CAD build for the part. Positions are in the model's coordinates, mm. A direction names the side the tool comes from. Coordinates: 2 decimals unless noted, no trailing zeros. Order: outer loops, then holes, each group sorted by start corner. A loop starts at its lowest first (then second) coordinate and runs counter-clockwise, first axis right, second up. Notation, with made-up numbers: (-11.75, -37) - (45.25, -37) arc R15 cw to (45.25, -31) - close; hole circle Ø3 at (80.25, 57). An arc over 180 degrees is marked (long way). Write each question's results on one line, items separated by ' | '. Start each with the question number.
Q1. Pin check, flat tips, straight feed: P1, Ø4, axis at x = 12, z = 5, coming from the +Y side; P2, Ø3.5, axis at x = 2, y = 20, coming from the +Z side; P3, Ø6, axis at x = -1, y = 26.5, coming from the -Z side; P4, Ø5, axis at x = -20, y = -1.5, coming from the -Z side. Stop position of each tip, or through.
Q2. Band-saw the part on B-B, the plane z = 2.75. Write the cut outline in (x, y).
Q3. Pull direction X, two halves, no side cores. Call faces 1 (the flat face through (15.968, -2.936, 6.726)), 2 (the flat face through (10.597, -12.391, 6.726)), 3 (the flat face through (-4.28, 25.19, 3.52)): released by +X, released by -X, zero draft, split by the parting line, or undercut.
Q4. Wall check: probe 1 along Y at (x, z) = (0, 1.5); probe 2 along Y at (x, z) = (6, 5.5); probe 3 along X at (y, z) = (-15, 5). Give the ranges that are in metal, low to high.
Q5. Which spindle directions (+Z, -Z, +X, -X, +Y, -Y) get a long thin tool onto all of the face, cutting with end or side? Do faces 4 (the flat face through (11, 2, 0)), 5 (the flat face through (-19.677, -16.304, 3.517)), 6 (the flat face through (4.304, 24.995, 3.517)), 7 (the flat face through (16.03, -2.98, 0.38)), 8 (the flat face through (-16.03, -2.98, 6.73)). Say none if no direction does.
Q6. Band-saw the part on C-C, the plane y = -9. Write the cut outline in (x, z), then the cut area to 3 significant figures.
Q7. Band-saw the part on D-D, the plane x = -7. Write the cut outline in (y, z), then the cut area to 3 significant figures.
Q8. Band-saw the part on A-A, the plane x = 0. Write the cut outline in (y, z).
```python
from build123d import *

# Parameters (mm, degrees)
F0_R     = 10.922
F1_DEPTH = 7.112
F2_DEPTH = 6.35
F3_DEPTH = 0.762
F4_DEPTH = 7.112


with BuildPart() as f1:
    # F0 (on Top) → F1 (new body)
    with BuildSketch(Plane.XY):
        with BuildLine():
            Line((-5.7560840378, 12.6157379826), (-5.1183423957, 18.0540294813))
            Line((-5.1183423957, 18.0540294813), (-9.9884684203, 9.6187237673))
            ThreePointArc((-9.9884684203, 9.6187237673), (-8.0136294261, 11.3168499026), (-5.7560840378, 12.6157379826))
        make_face()
        with BuildLine():
            ThreePointArc((5.7560840378, 12.6157379826), (0, 13.8668434871), (-5.7560840378, 12.6157379826))
            ThreePointArc((-5.7560840378, 12.6157379826), (-8.0136294261, 11.3168499026), (-9.9884684203, 9.6187237673))
            Line((-9.9884684203, 9.6187237673), (-13.3242933447, 3.8409055132))
            ThreePointArc((-13.3242933447, 3.8409055132), (-13.8074942195, 1.2815817082), (-13.8035915993, -1.3229539883))
            ThreePointArc((-13.8035915993, -1.3229539883), (-12.0090387301, -6.9334217436), (-8.0475075615, -11.2927839943))
            ThreePointArc((-8.0475075615, -11.2927839943), (-5.7938647934, -12.5984316108), (-3.3358249243, -13.4596292806))
            Line((-3.3358249243, -13.4596292806), (3.3358249243, -13.4596292806))
            ThreePointArc((3.3358249243, -13.4596292806), (5.7938647934, -12.5984316108), (8.0475075615, -11.2927839943))
            ThreePointArc((8.0475075615, -11.2927839943), (12.0090387301, -6.9334217436), (13.8035915993, -1.3229539883))
            ThreePointArc((13.8035915993, -1.3229539883), (13.8510214888, -0.6622325982), (13.8668434871, 0))
            ThreePointArc((13.8668434871, 0), (13.730536018, 1.9395177119), (13.3242933447, 3.8409055132))
            Line((13.3242933447, 3.8409055132), (9.9884684203, 9.6187237673))
            ThreePointArc((9.9884684203, 9.6187237673), (8.0136294261, 11.3168499026), (5.7560840378, 12.6157379826))
        make_face()
        Circle(F0_R, mode=Mode.SUBTRACT)
        with BuildLine():
            Line((5.1183423957, 18.0540294813), (5.7560840378, 12.6157379826))
            ThreePointArc((5.7560840378, 12.6157379826), (8.0136294261, 11.3168499026), (9.9884684203, 9.6187237673))
            Line((9.9884684203, 9.6187237673), (5.1183423957, 18.0540294813))
        make_face()
        with BuildLine():
            ThreePointArc((-13.8035915993, -1.3229539883), (-13.8074942195, 1.2815817082), (-13.3242933447, 3.8409055132))
            Line((-13.3242933447, 3.8409055132), (-18.1944193693, -4.5944002008))
            Line((-18.1944193693, -4.5944002008), (-13.8035915993, -1.3229539883))
        make_face()
        with BuildLine():
            Line((18.1944193693, -4.5944002008), (13.3242933447, 3.8409055132))
            ThreePointArc((13.3242933447, 3.8409055132), (13.730536018, 1.9395177119), (13.8668434871, 0))
            ThreePointArc((13.8668434871, 0), (13.8510214888, -0.6622325982), (13.8035915993, -1.3229539883))
            Line((13.8035915993, -1.3229539883), (18.1944193693, -4.5944002008))
        make_face()
        with BuildLine():
            ThreePointArc((8.0475075615, -11.2927839943), (5.7938647934, -12.5984316108), (3.3358249243, -13.4596292806))
            Line((3.3358249243, -13.4596292806), (13.0760769737, -13.4596292806))
            Line((13.0760769737, -13.4596292806), (8.0475075615, -11.2927839943))
        make_face()
    extrude(amount=F1_DEPTH)

    # F0 (on Top) → F2 (join)
    with BuildSketch(Plane.XY):
        with BuildLine():
            ThreePointArc((-8.0475075615, -11.2927839943), (-12.0090387301, -6.9334217436), (-13.8035915993, -1.3229539883))
            Line((-13.8035915993, -1.3229539883), (-18.1944193693, -4.5944002008))
            Line((-18.1944193693, -4.5944002008), (-29.5624734591, -13.0643241977))
            Line((-29.5624734591, -13.0643241977), (-26.095273368, -19.0696909155))
            Line((-26.095273368, -19.0696909155), (-13.0760769737, -13.4596292806))
            Line((-13.0760769737, -13.4596292806), (-8.0475075615, -11.2927839943))
        make_face()
        with BuildLine():
            Line((-3.4672000911, 32.1340151131), (-5.1183423957, 18.0540294813))
            Line((-5.1183423957, 18.0540294813), (-5.7560840378, 12.6157379826))
            ThreePointArc((-5.7560840378, 12.6157379826), (0, 13.8668434871), (5.7560840378, 12.6157379826))
            Line((5.7560840378, 12.6157379826), (5.1183423957, 18.0540294813))
            Line((5.1183423957, 18.0540294813), (3.4672000911, 32.1340151131))
            Line((3.4672000911, 32.1340151131), (-3.4672000911, 32.1340151131))
        make_face()
        with BuildLine():
            Line((29.5624734591, -13.0643241977), (18.1944193693, -4.5944002008))
            Line((18.1944193693, -4.5944002008), (13.8035915993, -1.3229539883))
            ThreePointArc((13.8035915993, -1.3229539883), (12.0090387301, -6.9334217436), (8.0475075615, -11.2927839943))
            Line((8.0475075615, -11.2927839943), (13.0760769737, -13.4596292806))
            Line((13.0760769737, -13.4596292806), (26.095273368, -19.0696909155))
            Line((26.095273368, -19.0696909155), (29.5624734591, -13.0643241977))
        make_face()
    extrude(amount=F2_DEPTH)

    # F0 (on Top) → F3 (cut)
    with BuildSketch(Plane.XY):
        with BuildLine():
            Line((29.5624734591, -13.0643241977), (18.1944193693, -4.5944002008))
            Line((18.1944193693, -4.5944002008), (13.8035915993, -1.3229539883))
            ThreePointArc((13.8035915993, -1.3229539883), (12.0090387301, -6.9334217436), (8.0475075615, -11.2927839943))
            Line((8.0475075615, -11.2927839943), (13.0760769737, -13.4596292806))
            Line((13.0760769737, -13.4596292806), (26.095273368, -19.0696909155))
            Line((26.095273368, -19.0696909155), (29.5624734591, -13.0643241977))
        make_face()
        with BuildLine():
            Line((-3.4672000911, 32.1340151131), (-5.1183423957, 18.0540294813))
            Line((-5.1183423957, 18.0540294813), (-5.7560840378, 12.6157379826))
            ThreePointArc((-5.7560840378, 12.6157379826), (0, 13.8668434871), (5.7560840378, 12.6157379826))
            Line((5.7560840378, 12.6157379826), (5.1183423957, 18.0540294813))
            Line((5.1183423957, 18.0540294813), (3.4672000911, 32.1340151131))
            Line((3.4672000911, 32.1340151131), (-3.4672000911, 32.1340151131))
        make_face()
        with BuildLine():
            ThreePointArc((-8.0475075615, -11.2927839943), (-12.0090387301, -6.9334217436), (-13.8035915993, -1.3229539883))
            Line((-13.8035915993, -1.3229539883), (-18.1944193693, -4.5944002008))
            Line((-18.1944193693, -4.5944002008), (-29.5624734591, -13.0643241977))
            Line((-29.5624734591, -13.0643241977), (-26.095273368, -19.0696909155))
            Line((-26.095273368, -19.0696909155), (-13.0760769737, -13.4596292806))
            Line((-13.0760769737, -13.4596292806), (-8.0475075615, -11.2927839943))
        make_face()
    extrude(amount=F3_DEPTH, mode=Mode.SUBTRACT)

    # F0 (on Top) → F4 (join)
    with BuildSketch(Plane.XY):
        with BuildLine():
            ThreePointArc((-3.3358249243, -13.4596292806), (-5.7938647934, -12.5984316108), (-8.0475075615, -11.2927839943))
            Line((-8.0475075615, -11.2927839943), (-13.0760769737, -13.4596292806))
            Line((-13.0760769737, -13.4596292806), (-3.3358249243, -13.4596292806))
        make_face()
    extrude(amount=F4_DEPTH)


solid = f1.part
```
Results below:
1) P1: stops at y = 9.6 | P2: stops at z = 6.35 | P3: stops at z = 0.76 | P4: passes through
2) outline: (-29.56, -13.06) - (-26.1, -19.07) - (-13.08, -13.46) - (13.08, -13.46) - (26.1, -19.07) - (29.56, -13.06) - (18.19, -4.59) - (5.12, 18.05) - (3.47, 32.13) - (-3.47, 32.13) - (-5.12, 18.05) - (-18.19, -4.59) - close; hole circle Ø21.84 at (0, 0)
3) face 1: undercut | face 2: released by +X | face 3: released by -X
4) probe 1: y = -13.46 to -10.92, 10.92 to 32.13 | probe 2: y = -13.46 to -9.13, 9.13 to 16.53 | probe 3: x = -28.44 to -16.65, 16.65 to 28.44
5) face 4: -Z, +X, -X, +Y, -Y | face 5: +Z, -Z, -Y | face 6: +Z, -Z, +X, +Y | face 7: -Z, -Y | face 8: +Z, -Y
6) outline: (-24.11, 0.76) - (-10.55, 0.76) - (-10.55, 0) - (-6.19, 0) - (-6.19, 7.11) - (-10.55, 7.11) - (-10.55, 6.35) - (-24.11, 6.35) - close; (6.19, 0) - (10.55, 0) - (10.55, 0.76) - (24.11, 0.76) - (24.11, 6.35) - (10.55, 6.35) - (10.55, 7.11) - (6.19, 7.11) - close | area: 214 mm²
7) outline: (-13.46, 0) - (-8.38, 0) - (-8.38, 7.11) - (-13.46, 7.11) - close; (8.38, 0) - (14.79, 0) - (14.79, 7.11) - (8.38, 7.11) - close | area: 81.7 mm²
8) outline: (-13.46, 0) - (-10.92, 0) - (-10.92, 7.11) - (-13.46, 7.11) - close; (10.92, 0) - (13.87, 0) - (13.87, 0.76) - (32.13, 0.76) - (32.13, 6.35) - (13.87, 6.35) - (13.87, 7.11) - (10.92, 7.11) - close
